from build123d import *

# Parameters (mm, degrees)
SKETCH1_W           = 50.8
SKETCH1_H           = 546.1
BOSS_EXTRUDE1_DEPTH = 50.8
SKETCH2_W           = 44.45
SKETCH2_H           = 44.45
CUT_EXTRUDE1_DEPTH  = 547.1
SKETCH4_R           = 16.7005
SKETCH4_R_2         = 3.302
CUT_EXTRUDE2_DEPTH  = 51.8


with BuildPart() as part:
    # Sketch1 → Boss-Extrude1 (new body)
    with BuildSketch(Plane(origin=(0, 0, 0), x_dir=(0, 0, -1), z_dir=(1, 0, 0))):
        Rectangle(SKETCH1_W, SKETCH1_H)
    extrude(amount=BOSS_EXTRUDE1_DEPTH)

    # Sketch2 → Cut-Extrude1 (cut, through all)
    with BuildSketch(Plane(origin=(0, 273.05, 0), x_dir=(1, 0, 0), z_dir=(0, 1, 0))):
        with Locations((25.4, 0)):
            Rectangle(SKETCH2_W, SKETCH2_H)
    extrude(amount=-CUT_EXTRUDE1_DEPTH, mode=Mode.SUBTRACT)

    # Sketch4 → Cut-Extrude2 (cut, through all)
    with BuildSketch(Plane(origin=(50.8, 0, 0), x_dir=(0, 0, -1), z_dir=(1, 0, 0))):
        with Locations((0, -133.35)):
            Circle(SKETCH4_R)
        with Locations((0, -82.598640474)):
            Circle(SKETCH4_R_2)
    extrude(amount=-CUT_EXTRUDE2_DEPTH, mode=Mode.SUBTRACT)


solid = part.part
Model file for the job. Use its own axes, mm. A direction names the side the tool comes from. Give positions to 0.01 mm unless a question says otherwise; leave off trailing zeros. Write each loop counter-clockwise with the first axis right and the second up, starting at its lowest first coordinate (ties: lowest second). Pieces come first, ordered by that corner, then holes. Notation, with made-up numbers: (-35.75, 72.5) - (20.25, 72.5) arc R31 ccw to (20.25, 99.5) - close; hole circle Ø4 at (65.5, 49). An arc over 180 degrees is marked (long way). Answer as CSV lines item,"result".
1. Two-plate mould, pull along X, no slides. Class faces 1 (the face through (47.625, 4, 0)), 2 (the face through (0, 4, 0)), 3 (the face through (50.8, 4, 0)), 4 (the face through (1.61, -116.79, 2.17)): +X half, -X half, draft (parallel to the pull), parting line (faces both ways), or undercut.
Responses:
face 1,"undercut"
face 2,"-X half"
face 3,"+X half"
face 4,"draft"
2. Pin check, flat tip, straight feed: pin 1 (8 mm diameter, centred on y = 103, z = 6.5, fed in from -X). Stop position of the tip, or through.
Responses:
pin 1,"stops at x = 0"
3. Drill centre lines: L1, parallel to Y at x = 1, z = 0; L2, parallel to Z at x = 5.5, y = -66 (3 decimals); L3, parallel to X at y = 101.5, z = -16.5 (3 decimals). Where is each one in solid material? Low to high. Write a range as [from, to].
Responses:
L1,"y = [-273.05, -150.05], [-116.65, -85.9], [-79.3, 273.05]"
L2,"z = [-25.4, -22.225], [22.225, 25.4]"
L3,"x = [0, 3.175], [47.625, 50.8]"
4. 3-axis set-ups, long thin cutter, end or side, ignore diameter. For faces 5 (the face through (3.175, 4, 0)), 6 (the face through (25, -4, -25.4)): which of +Z, -Z, +X, -X, +Y, -Y reach the whole face in a straight line?
Responses:
face 5,"+Y, -Y"
face 6,"-Z, +X, -X, +Y, -Y"
5. Band-saw the part on D-D (y = -133.35). Write the cut outline in (x, z) (1 decimal), and give its area (3 significant figures).
Responses:
outline,"(0, -25.4) - (50.8, -25.4) - (50.8, -16.7) - (47.6, -16.7) - (47.6, -22.2) - (3.2, -22.2) - (3.2, -16.7) - (0, -16.7) - close; (0, 16.7) - (3.2, 16.7) - (3.2, 22.2) - (47.6, 22.2) - (47.6, 16.7) - (50.8, 16.7) - (50.8, 25.4) - (0, 25.4) - close"
area,"393 mm2"
6. Band-saw the part on A-A (x = 18). Write the cut outline in (y, z) (3 decimals), and give its area (3 significant figures).
Responses:
outline,"(-273.05, -25.4) - (273.05, -25.4) - (273.05, -22.225) - (-273.05, -22.225) - close; (-273.05, 22.225) - (273.05, 22.225) - (273.05, 25.4) - (-273.05, 25.4) - close"
area,"3,470 mm2"
7. Band-saw the part on C-C (z = -11). Write the cut outline in (x, y) (3 decimals), and give its area (3 significant figures).
Responses:
outline,"(0, -273.05) - (3.175, -273.05) - (3.175, -145.916) - (0, -145.916) - close; (0, -120.784) - (3.175, -120.784) - (3.175, 273.05) - (0, 273.05) - close; (47.625, -273.05) - (50.8, -273.05) - (50.8, -145.916) - (47.625, -145.916) - close; (47.625, -120.784) - (50.8, -120.784) - (50.8, 273.05) - (47.625, 273.05) - close"
area,"3,310 mm2"
8. Band-saw the part on B-B (y = -214). Write the cut outline in (x, z) (3 decimals).
Responses:
outline,"(0, -25.4) - (50.8, -25.4) - (50.8, 25.4) - (0, 25.4) - close; hole (3.175, -22.225) - (47.625, -22.225) - (47.625, 22.225) - (3.175, 22.225) - close"
